Answer from the drawing. Dimensions are ordinates in mm from the lowest x, y and z of the part. A direction names the side the tool comes from. Coordinates: 2 decimals unless noted, no trailing zeros. Order: outer loops, then holes, each group sorted by start corner. A loop starts at its lowest first (then second) coordinate and runs counter-clockwise, first axis right, second up. Notation, with made-up numbers: M 78,63.25 L 93,63.25 A7 ccw 93,68.25 Z; hole C 36.25,89.25 d10. An arc over 180 degrees is marked long. Write each question's results on one line, items separated by ' | '.
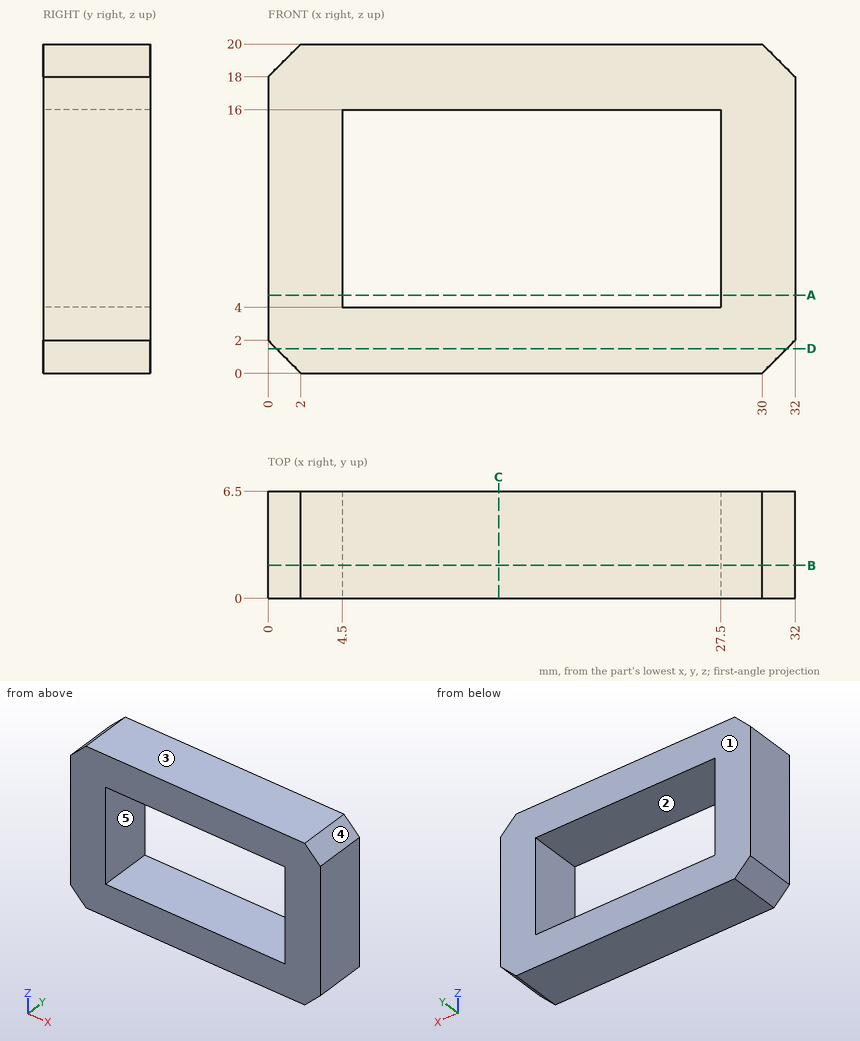
(1) The part is cut by section A-A, the plane z = 4.75. Write down the section's boundary in (x, y), then the cut area to 3 significant figures.
Conclusion:
outline: M 0,0 L 4.5,0 L 4.5,6.5 L 0,6.5 Z; M 27.5,0 L 32,0 L 32,6.5 L 27.5,6.5 Z | area: 58.5 mm²
(2) Straight lines are drawn through the part: line 1 (Z direction, x = 19.5, y = 4.75); line 2 (X direction, y = 5.75, z = 5.5); line 3 (X direction, y = 0.5, z = 1.25). For each, find the intervals that lie inside material, in ascending order.
Conclusion:
line 1: 0 to 4, 16 to 20 | line 2: 0 to 4.5, 27.5 to 32 | line 3: 0.75 to 31.25
(3) The part is cut by section C-C, the plane x = 14. Write down the section's boundary in (y, z), then the cut area to 3 significant figures.
Conclusion:
outline: M 0,0 L 6.5,0 L 6.5,4 L 0,4 Z; M 0,16 L 6.5,16 L 6.5,20 L 0,20 Z | area: 52.0 mm²
(4) The mould has two halves that part along X. Classify the marked faces 3, 4 and 5: pulls with the +X half, pulls with the -X half, needs draft (parallel to the pull), parting line crosses it, or undercut.
Conclusion:
face 3: needs draft | face 4: pulls with the +X half | face 5: undercut
(5) For the marked faces 1 and 2, determine the directions among +Z, -Z, +X, -X, +Y, -Y from which every point of the face is accessible in a straight line to the end or side of a thin tool.
Conclusion:
face 1: +Z, -Z, +X, -X, +Y | face 2: +Y, -Y
(6) The part is cut by section B-B, the plane y = 2. Write down the section's boundary in (x, z), then the cut area to 3 significant figures.
Conclusion:
outline: M 0,2 L 2,0 L 30,0 L 32,2 L 32,18 L 30,20 L 2,20 L 0,18 Z; hole M 4.5,4 L 27.5,4 L 27.5,16 L 4.5,16 Z | area: 356 mm²
(7) The part is cut by section D-D, the plane z = 1.5. Write down the section's boundary in (x, y), then the cut area to 4 significant figures.
Conclusion:
outline: M 0.5,0 L 31.5,0 L 31.5,6.5 L 0.5,6.5 Z | area: 201.5 mm²
